Check sheet for the modelled part. Datum: model origin and axes. Units: mm. Face numbers are marked on the shaded views. A direction names the side the tool comes from. Give positions to 0.01 mm unless a question says otherwise; leave off trailing zeros. Write each loop counter-clockwise with the first axis right and the second up, starting at its lowest first coordinate (ties: lowest second). Pieces come first, ordered by that corner, then holes. Notation, with made-up numbers: (-20.5, 23.5) -> (30.5, 23.5) arc R16 ccw to (30.5, 53.5) -> close; hole circle Ø5 at (43.5, -36). An arc over 180 degrees is marked (long way). Return JSON: item names as keys, results as strings.
from build123d import *

# Parameters (mm, degrees)
F0_W      = 7
F0_H      = 7
F1_DEPTH  = 3.5
F2_R      = 3.5
F2_R_2    = 1.75
F3_DEPTH  = 6
F4_R      = 3.5
F4_R_2    = 1.75
F5_DEPTH  = 6
F6_R      = 3.5
F6_R_2    = 1.75
F7_DEPTH  = 6
F8_R      = 3.5
F8_R_2    = 1.75
F9_DEPTH  = 6
F10_R     = 3.5
F10_R_2   = 1.75
F11_DEPTH = 6
F12_R     = 3.5
F12_R_2   = 1.75
F13_DEPTH = 6


with BuildPart() as f1:
    # F0 (on Front) → F1 (new body, symmetric)
    with BuildSketch(Plane.XZ):
        Rectangle(F0_W, F0_H)
    extrude(amount=F1_DEPTH, both=True)

    # F2 (on face) → F3 (join)
    with BuildSketch(Plane.XZ.offset(3.5)):
        Circle(F2_R)
        Circle(F2_R_2, mode=Mode.SUBTRACT)
    extrude(amount=F3_DEPTH)

    # F4 (on face) → F5 (join)
    with BuildSketch(Plane(origin=(0, 0, -3.5), x_dir=(1, 0, 0), z_dir=(0, 0, -1))):
        Circle(F4_R)
        Circle(F4_R_2, mode=Mode.SUBTRACT)
    extrude(amount=F5_DEPTH)

    # F6 (on face) → F7 (join)
    with BuildSketch(Plane(origin=(0, 3.5, 0), x_dir=(-1, 0, 0), z_dir=(0, 1, 0))):
        Circle(F6_R)
        Circle(F6_R_2, mode=Mode.SUBTRACT)
    extrude(amount=F7_DEPTH)

    # F8 (on face) → F9 (join)
    with BuildSketch(Plane.XY.offset(3.5)):
        Circle(F8_R)
        Circle(F8_R_2, mode=Mode.SUBTRACT)
    extrude(amount=F9_DEPTH)

    # F10 (on face) → F11 (join)
    with BuildSketch(Plane(origin=(-3.5, 0, 0), x_dir=(0, -1, 0), z_dir=(-1, 0, 0))):
        Circle(F10_R)
        Circle(F10_R_2, mode=Mode.SUBTRACT)
    extrude(amount=F11_DEPTH)

    # F12 (on face) → F13 (join)
    with BuildSketch(Plane.YZ.offset(3.5)):
        Circle(F12_R)
        Circle(F12_R_2, mode=Mode.SUBTRACT)
    extrude(amount=F13_DEPTH)


solid = f1.part
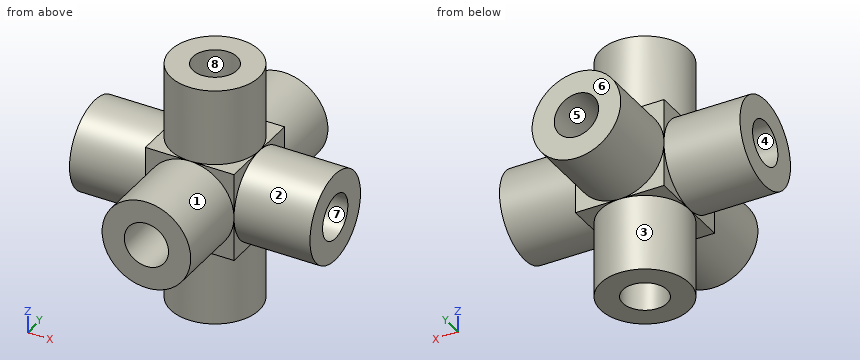
(1) Depth check by flat-ended pin: pin 1 Ø6 at (x, y) = (-6, -3.5) entering from +Z; pin 2 Ø2 at (y, z) = (0, 0) entering from -X; pin 3 Ø6 at (y, z) = (-7, -4.5) entering from +X. Enter the tip coordinate at first touch or a pass-through.
Reply:
{"pin 1": "z = 3.5", "pin 2": "x = -3.5", "pin 3": "x = 3.16"}
(2) Set-up check for the marked faces 1, 2, 3 and 4: record each of +Z, -Z, +X, -X, +Y, -Y from which the full face is reachable in a straight line by a thin tool's end or side.
Reply:
{"face 1": "-Y", "face 2": "+X", "face 3": "-Z", "face 4": "-X"}
(3) Cross-section at D-D on y = 2.25. Enter the section's corners in (x, z).
Reply:
{"outline": "(-9.5, -2.68) -> (-3.5, -2.68) -> (-3.5, -3.5) -> (-2.68, -3.5) -> (-2.68, -9.5) -> (2.68, -9.5) -> (2.68, -3.5) -> (3.5, -3.5) -> (3.5, -2.68) -> (9.5, -2.68) -> (9.5, 2.68) -> (3.5, 2.68) -> (3.5, 3.5) -> (2.68, 3.5) -> (2.68, 9.5) -> (-2.68, 9.5) -> (-2.68, 3.5) -> (-3.5, 3.5) -> (-3.5, 2.68) -> (-9.5, 2.68) -> close"}
(4) Release check for a two-part mould opening along Y. For the marked faces 5, 6, 7 and 8 record: pulls with the +Y half, pulls with the -Y half, needs draft (parallel to the pull), parting line crosses it, or undercut.
Reply:
{"face 5": "needs draft", "face 6": "pulls with the +Y half", "face 7": "undercut", "face 8": "undercut"}
(5) Cross-section at A-A on z = -6.5. Enter the section's corners in (x, y), then the cut area to 3 significant figures.
Reply:
{"outline": "circle Ø7 at (0, 0); hole circle Ø3.5 at (0, 0)", "area": "28.9 mm^2"}
(6) Thickness scan on L1, parallel to Y at x = 0, z = -5.55. Record the ranges inside material, lowest first.
Reply:
{"L1": "-3.5 to -1.75, 1.75 to 3.5"}
(7) Cross-section at C-C on z = 2.75. Enter the section's corners in (x, y), then the cut area to 3 significant figures.
Reply:
{"outline": "(-9.5, -2.17) -> (-3.5, -2.17) -> (-3.5, -3.5) -> (-2.17, -3.5) -> (-2.17, -9.5) -> (2.17, -9.5) -> (2.17, -3.5) -> (3.5, -3.5) -> (3.5, -2.17) -> (9.5, -2.17) -> (9.5, 2.17) -> (3.5, 2.17) -> (3.5, 3.5) -> (2.17, 3.5) -> (2.17, 9.5) -> (-2.17, 9.5) -> (-2.17, 3.5) -> (-3.5, 3.5) -> (-3.5, 2.17) -> (-9.5, 2.17) -> close", "area": "153 mm^2"}
